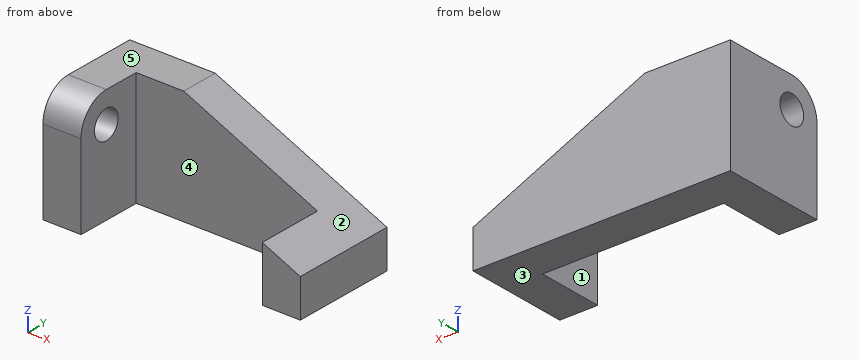
```python
from build123d import *

# Parameters (mm, degrees)
BOSS_EXTRUDE3_DEPTH     = 60
CUT_EXTRUDE1_DEPTH      = 97.950548376
CUT_EXTRUDE1_DEPTH_BACK = 97.950548376
FILLET3_R               = 16
SKETCH7_R               = 7.5
CUT_EXTRUDE2_DEPTH      = 100


with BuildPart() as part:
    # Sketch3 → Boss-Extrude3 (new body)
    with BuildSketch(Plane.XY):
        Polygon((-47.6343761, -55), (-47.6343761, -20), (47.6343761, -20), (47.6343761, -55), (67.6343761, -55), (67.6343761, 0), (-67.6343761, 0), (-67.6343761, -55), align=None)
    extrude(amount=BOSS_EXTRUDE3_DEPTH)

    # Sketch4 → Cut-Extrude1 (cut, two sides: drawn at the far end of the back side and taken through both)
    with BuildSketch(Plane.XZ.offset(20).offset(-CUT_EXTRUDE1_DEPTH_BACK)):
        Polygon((-22.6343761, 60), (67.6343761, 60), (67.6343761, 20), align=None)
    extrude(amount=CUT_EXTRUDE1_DEPTH + CUT_EXTRUDE1_DEPTH_BACK, mode=Mode.SUBTRACT)

    # Fillet3
    fillet3_edges = [part.edges().sort_by_distance(p)[0] for p in [
        (-57.6343761, -55, 60),
    ]]
    fillet(fillet3_edges, radius=FILLET3_R)

    # Sketch7 → Cut-Extrude2 (cut)
    with BuildSketch(Plane(origin=(-47.6343761, 0, 0), x_dir=(0, 0, -1), z_dir=(1, 0, 0))):
        with Locations((-44, -39)):
            Circle(SKETCH7_R)
    extrude(amount=-CUT_EXTRUDE2_DEPTH, mode=Mode.SUBTRACT)


solid = part.part
```
The listing builds one solid part. Answer for the finished solid, in the listing's coordinates (mm). Face numbers are marked on the shaded views. A direction names the side the tool comes from. Coordinates: 2 decimals unless noted, no trailing zeros. Write each loop counter-clockwise with the first axis right and the second up, starting at its lowest first coordinate (ties: lowest second). Pieces come first, ordered by that corner, then holes. Notation, with made-up numbers: (-20.5, 38) - (26.5, 38) arc R18 ccw to (26.5, 49) - close; hole circle Ø3 at (0, 78). An arc over 180 degrees is marked (long way). Return JSON: item names as keys, results as strings. Group by question number.
1. Which of the six approach directions +Z, -Z, +X, -X, +Y, -Y give full straight-line access (tool end or side, diameter ignored) to the marked faces 4 and 5?
2. A cutting plane is placed at D-D, the plane x = -42. Determine the outline of the cut face in (y, z), plus the area to 3 significant figures.
3. Determine the mould class of the marked faces 1, 2 and 3 for opening direction X: released by +X, released by -X, zero draft, split by the parting line, or undercut.
4. Straight lines are drawn through the part: L1, parallel to Y at x = -57, z = 44; L2, parallel to X at y = -29.5, z = 8; L3, parallel to X at y = -40, z = 55. For each, find the intervals that lie inside material, in ascending order.
5. A cutting plane is placed at A-A, the plane y = -30. Determine the outline of the cut face in (x, z), plus the area to 3 significant figures.
6. A cutting plane is placed at B-B, the plane z = 21.5. Determine the outline of the cut face in (x, y).
7. Given pin 1 (2 mm diameter, centred on y = -26.5, z = 39.5, fed in from +X); pin 2 (6 mm diameter, centred on x = -14, z = 22.5, fed in from +Y); pin 3 (8 mm diameter, centred on x = 23.5, z = 39, fed in from -Y), each flat-ended and moving along its own axis, determine where each tip first touches the part or whether it passes through.
8. A cutting plane is placed at C-C, the plane y = -5. Determine the outline of the cut face in (x, z).
Ans:
{
 "1": {"face 4": "+Z, -Z, -Y", "face 5": "+Z, +X, -X, +Y, -Y"},
 "2": {"outline": "(-20, 0) - (0, 0) - (0, 60) - (-20, 60) - close", "area": "1,200 mm²"},
 "3": {"face 1": "undercut", "face 2": "released by +X", "face 3": "zero draft"},
 "4": {"L1": "-55 to -46.5, -31.5 to 0", "L2": "-67.63 to -47.63, 47.63 to 67.63", "L3": "-67.63 to -47.63"},
 "5": {"outline": "(-67.63, 0) - (-47.63, 0) - (-47.63, 60) - (-67.63, 60) - close; (47.63, 0) - (67.63, 0) - (67.63, 20) - (47.63, 28.86) - close", "area": "1,690 mm²"},
 "6": {"outline": "(-67.63, -55) - (-47.63, -55) - (-47.63, -20) - (47.63, -20) - (47.63, -55) - (64.25, -55) - (64.25, 0) - (-67.63, 0) - close"},
 "7": {"pin 1": "x = -47.63", "pin 2": "y = 0", "pin 3": "y = -20"},
 "8": {"outline": "(-67.63, 0) - (67.63, 0) - (67.63, 20) - (-22.63, 60) - (-67.63, 60) - close"}
}
